```python
from build123d import *

# Parameters (mm, degrees)
SKETCH_4_W      = 115
SKETCH_4_H      = 145
EXTRUDE_1_DEPTH = 2
SKETCH_5_W      = 16
SKETCH_5_H      = 2
EXTRUDE_2_DEPTH = 2
SKETCH_6_W      = 21
SKETCH_6_H      = 2
EXTRUDE_3_DEPTH = 4.5
EXTRUDE_START   = -115
SKETCH_6_2_W    = 21
SKETCH_6_2_H    = 2
EXTRUDE_4_DEPTH = 6.5
EXTRUDE_START_2 = -2.2
EXTRUDE_5_DEPTH = 142.8


with BuildPart() as part:
    # 草图4 → 凸台-拉伸1 (new body)
    with BuildSketch(Plane(origin=(0, 0, 0), x_dir=(1, 0, 0), z_dir=(0, 1, 0))):
        Rectangle(SKETCH_4_W, SKETCH_4_H)
    extrude(amount=EXTRUDE_1_DEPTH)

    # 草图5 → 凸台-拉伸2 (add)
    with BuildSketch(Plane(origin=(0, 0, -72.5), x_dir=(-1, 0, 0), z_dir=(0, 0, -1))):
        with Locations((-49.5, 1)):
            Rectangle(SKETCH_5_W, SKETCH_5_H)
        with Locations((-16.5, 1)):
            Rectangle(SKETCH_5_W, SKETCH_5_H)
        with Locations((16.5, 1)):
            Rectangle(SKETCH_5_W, SKETCH_5_H)
        with Locations((49.5, 1)):
            Rectangle(SKETCH_5_W, SKETCH_5_H)
    extrude(amount=EXTRUDE_2_DEPTH)

    # 草图6 → 凸台-拉伸3 (add)
    with BuildSketch(Plane.ZY.offset(57.5)):
        with Locations((-43, 1)):
            Rectangle(SKETCH_6_W, SKETCH_6_H)
        with Locations((-1, 1)):
            Rectangle(SKETCH_6_W, SKETCH_6_H)
        with Locations((41, 1)):
            Rectangle(SKETCH_6_W, SKETCH_6_H)
    extrude(amount=EXTRUDE_3_DEPTH)

    # 草图6<2> → 凸台-拉伸4 (add)
    with BuildSketch(Plane.ZY.offset(57.5).offset(EXTRUDE_START)):
        with Locations((-43, 1)):
            Rectangle(SKETCH_6_2_W, SKETCH_6_2_H)
        with Locations((-1, 1)):
            Rectangle(SKETCH_6_2_W, SKETCH_6_2_H)
        with Locations((41, 1)):
            Rectangle(SKETCH_6_2_W, SKETCH_6_2_H)
    extrude(amount=-EXTRUDE_4_DEPTH)

    # 草图8 → 凸台-拉伸5 (add)
    with BuildSketch(Plane.XY.offset(72.5).offset(EXTRUDE_START_2)):
        Polygon((-43.1, 3.8), (-41.3, 2), (-21.7, 2), (-19.9, 3.8), (-21.7, 3.8), (-41.3, 3.8), align=None)
        Polygon((21.7, 2), (41.3, 2), (43.1, 3.8), (41.3, 3.8), (21.7, 3.8), (19.9, 3.8), align=None)
    extrude(amount=-EXTRUDE_5_DEPTH)


solid = part.part
```
Check sheet for the modelled part. Datum: model origin and axes. Units: mm. Give positions to 0.01 mm unless a question says otherwise; leave off trailing zeros. Order: outer loops, then holes, each group sorted by start corner. A loop starts at its lowest first (then second) coordinate and runs counter-clockwise, first axis right, second up. Notation, with made-up numbers: (55.25, 8.25) -> (78.25, 8.25) arc R26 cw to (78.25, 31.25) -> close; hole circle Ø9 at (51, -14). An arc over 180 degrees is marked (long way). Return JSON: item names as keys, results as strings.
1. Cross-section at C-C, the plane z = 5. Record the cut outline in (x, y), plus the area to 3 significant figures.
From the geometry:
{"outline": "(-62, 0) -> (64, 0) -> (64, 2) -> (41.3, 2) -> (43.1, 3.8) -> (19.9, 3.8) -> (21.7, 2) -> (-21.7, 2) -> (-19.9, 3.8) -> (-43.1, 3.8) -> (-41.3, 2) -> (-62, 2) -> close", "area": "329 mm^2"}
2. Go/stop test with flat-tipped pins: P1, Ø1, axis at y = 0.5, z = -73.5, coming from the -X side; P2, Ø1, axis at x = 41.5, y = 3, coming from the +Z side; P3, Ø1, axis at x = 40, y = 1, coming from the -Z side; P4, Ø3, axis at x = 13, z = -13, coming from the -Y side. Record where each tip stops, or that it passes through.
From the geometry:
{"P1": "x = -57.5", "P2": "z = 70.3", "P3": "z = -72.5", "P4": "y = 0"}
3. Material ranges on probe 1 along Z at (x, y) = (36.5, 0.55); probe 2 along Y at (x, z) = (19, -18); probe 3 along X at (y, z) = (2.95, 40), recorded low to high. Write a range as [from, to].
From the geometry:
{"probe 1": "[-72.5, 72.5]", "probe 2": "[0, 2]", "probe 3": "[-42.25, -20.75], [20.75, 42.25]"}
4. Mould release check, pull along X, two halves, no side actions. Record for faces 1 (the flat face through (32, 3.8, 0)), 2 (the flat face through (2, 2, 0)): +X half, -X half, draft (parallel to the pull), parting line (faces both ways), or undercut.
From the geometry:
{"face 1": "draft", "face 2": "undercut"}
5. Cross-section at D-D, the plane z = 26. Record the cut outline in (x, y).
From the geometry:
{"outline": "(-57.5, 0) -> (57.5, 0) -> (57.5, 2) -> (41.3, 2) -> (43.1, 3.8) -> (19.9, 3.8) -> (21.7, 2) -> (-21.7, 2) -> (-19.9, 3.8) -> (-43.1, 3.8) -> (-41.3, 2) -> (-57.5, 2) -> close"}
6. Cross-section at B-B, the plane x = -39. Record the cut outline in (y, z), plus the area to 3 significant figures.
From the geometry:
{"outline": "(0, -72.5) -> (3.8, -72.5) -> (3.8, 70.3) -> (2, 70.3) -> (2, 72.5) -> (0, 72.5) -> close", "area": "547 mm^2"}
7. Cross-section at A-A, the plane y = 2.8. Record the cut outline in (x, z).
From the geometry:
{"outline": "(-42.1, -72.5) -> (-20.9, -72.5) -> (-20.9, 70.3) -> (-42.1, 70.3) -> close; (20.9, -72.5) -> (42.1, -72.5) -> (42.1, 70.3) -> (20.9, 70.3) -> close"}
